Could you check a few things on this model? Use its own coordinates, in mm. Give positions to 0.01 mm unless a question says otherwise; leave off trailing zeros. Order: outer loops, then holes, each group sorted by start corner. A loop starts at its lowest first (then second) coordinate and runs counter-clockwise, first axis right, second up. Notation, with made-up numbers: M -21,46.25 L -6,46.25 A14 cw -6,51.25 Z; hole C -14,80 d9. An arc over 180 degrees is marked long. Use a Markdown table: item, result. Add a question column.
Autodesk Inventor part; units mm, degrees
ref_plane "YZ Plane" through (0, 0, 0) normal (1, 0, 0) x (0, 1, 0)
ref_plane "XZ Plane" through (0, 0, 0) normal (0, 1, 0) x (-1, 0, 0)
ref_plane "XY Plane" through (0, 0, 0) normal (0, 0, 1) x (1, 0, 0)
sketch "Sketch1" plane through (0, 0, 0) normal (0, 1, 0) x (-1, 0, 0)
  line L0 (600, 0) -> (600, -30)
  arc A0 (529.3399, -125.599) -> (600, -30) centre (500, -30) ccw
  arc A1 (0, -205) -> (529.3399, -125.599) centre (0, 1599.1667) ccw
  line L1 (0, 191.6842) -> (0, -191.6842)
  arc A2 (0, -199) -> (527.5795, -119.8631) centre (0, 1599.1667) ccw
  arc A3 (527.5795, -119.8631) -> (594, -30) centre (500, -30) ccw
  line L2 (594, -30) -> (594, 0)
  line L3 (594, 0) -> (600, 0)
  line L4 (0, -199) -> (0, -205)
  point P0 (0, 0)
  point P1 (0, 0)
  point P2 (0, -202)
  point P3 (0, -163.7009)
  point P4 (0, -169.7009)
  dimension "d0" = 100
  dimension "d1" = 30
  dimension "d3" = 1804.1667
  dimension "d6" = 6
  dimension "d11" = 1188
  dimension "d12" = 205
revolve "Revolution1" add sketch "Sketch1" angle 360 about axis through (0, 0, 191.6842) along (0, 0, -1)
sketch "Sketch2" plane through (0, 0, 0) normal (0, 0, 1) x (1, 0, 0)
  circle A0 centre (0, 0) radius 45.5
  dimension "d8" = 91
extrude "Extrusion1" cut sketch "Sketch2" against normal through all
equation "\"d11\" = MAIN_filter_diam"
equation "\"MAIN_filter_diam\" = 1188"
equation "\"Disherd_head_hight\" = d12"
properties part number "PRS 940-02 dished head" material "Steel"
1) Please list where these lines run through material, in increasing order: line 1 (Y direction, x = 0, z = -6); line 2 (X direction, y = -101.5, z = -102); line 3 (X direction, y = 87.5, z = -94). Write a range as from..to.
2) We'd pull the mould along Y, two halves only. Please class faces 1 (the face through (581, 136, 0)), 2 (the face through (78.108, 594.894, -15.21)), 3 (the face through (77.327, -588.945, -14.79)): pulls with the +Y half, pulls with the -Y half, needs draft (parallel to the pull), parting line crosses it, or undercut.
3) For pin 1 (2 mm diameter, centred on x = 324, y = -440.5, fed in from +Z); pin 2 (4 mm diameter, centred on x = 376.5, y = 302, fed in from -Z) (3 decimals); pin 3 (4 mm diameter, centred on x = -107.5, y = 200, fed in from +Z), each with a flat end and sliding along its axis, tell me the tip position at first contact or that it passes through.
4) Suppose I cut it at A-A on z = -94.5. Please give me the cut outline in (x, y), and give its area (3 significant figures).
Values found:
| question | item | result |
|---|---|---|
| 1 | line 1 | y = -600..-594, 594..600 |
| 1 | line 2 | x = -560.28..-551.16, 551.16..560.28 |
| 1 | line 3 | x = -570.16..-562.08, 562.08..570.16 |
| 2 | face 1 | needs draft |
| 2 | face 2 | parting line crosses it |
| 2 | face 3 | undercut |
| 3 | pin 1 | stops at z = -110.93 |
| 3 | pin 2 | stops at z = -139.795 |
| 3 | pin 3 | stops at z = -184.35 |
| 4 | outline | C 0,0 d1152.84; hole C 0,0 d1136.76 |
| 4 | area | 28,900 mm^2 |
